Input: part model. Units: mm. Frame: model coordinates. Face numbers are marked on the shaded views. A direction names the side the tool comes from. Round coordinates to 2 decimals unless told otherwise and drop trailing zeros. Loops run counter-clockwise (first coordinate to the right, second up) from the corner with the lowest first, then second, coordinate; pieces in that order, holes last. Notation, with made-up numbers: M 84,46.25 L 98,46.25 A17 ccw 98,70.25 Z; hole C 35.5,47.5 d10. An arc over 180 degrees is marked long. Use one line per item in the form item = value. Start each with the question number.
Q1. Section query D-D, the plane y = 5.25. Output: boundary loops of the cut face in (x, z), and give its area (3 significant figures).
Q2. Mould query, pull axis Z, two halves, no side actions, for the marked faces 1, 2 and 3. Classes: pulls with the +Z half, pulls with the -Z half, needs draft (parallel to the pull), parting line crosses it, or undercut.
Q3. Section query A-A, the plane x = -13. Output: boundary loops of the cut face in (y, z), and give its area (3 significant figures).
Q4. Section query B-B, the plane z = 0. Output: boundary loops of the cut face in (x, y).
Q5. Access query for the marked faces 4, 5 and 6. Directions: +Z, -Z, +X, -X, +Y, -Y. A direction counts if a zero-diameter tool reaches every point of the face in a straight line with its end or side. Return the directions, or none.
Q6. Ray query, line 1 along Z through (x, y) = (-13.5, 1.25); line 2 along X through (y, z) = (-4.75, -0.75); line 3 along X through (y, z) = (-1.5, -1.25). Return the intervals inside material, ascending.
Q7. First-contact query: P1, Ø3, axis at x = -14, z = -0.5, coming from the -Y side; P2, Ø2, axis at y = 4.5, z = -4, coming from the +X side; P3, Ø1.5, axis at x = -4, y = 0.5, coming from the +Z side. Flat tips, straight axial feed; report the tip coordinate or a pass-through.
Q8. Section query C-C, the plane x = 8.5. Output: boundary loops of the cut face in (y, z), and give its area (3 significant figures).
Solid Edge part; units mm, degrees
sketch "Sketch1" plane through (10.8674, 0, 10.8674) normal (0, -1, 0) x (1, 0, 0)
  line L0 (-27.3674, -10.8674) -> (-27.3674, -4.3674)
  line L1 (-27.3674, -4.3674) -> (-19.3674, -4.3674)
  line L2 (-19.3674, -4.3674) -> (-19.3674, -6.4674)
  arc A0 (-19.3674, -6.4674) -> (-18.9674, -6.8674) centre (-18.9674, -6.4674) ccw
  line L3 (-18.9674, -6.8674) -> (5.6326, -6.8674)
  line L4 (5.6326, -6.8674) -> (5.6326, -10.8674)
revolve "RevolvedProtrusion1" add sketch "Sketch1" angle 360 about axis through (16.5, 0, 0) along (-1, 0, 0)
sketch "Sketch2" plane through (-16.5, 0, 0) normal (-1, 0, 0) x (0, 0, -1)
  line L0 (3.4641, 0) -> (1.7321, 3)
  line L1 (1.7321, 3) -> (-1.7321, 3)
  line L2 (-1.7321, 3) -> (-3.4641, 0)
  line L3 (-3.4641, 0) -> (-1.7321, -3)
  line L4 (-1.7321, -3) -> (1.7321, -3)
  line L5 (1.7321, -3) -> (3.4641, 0)
extrude "Cutout1" cut sketch "Sketch2" against normal blind 4
cosmetic_thread "Gänga" thread depth 20
properties material "Steel"
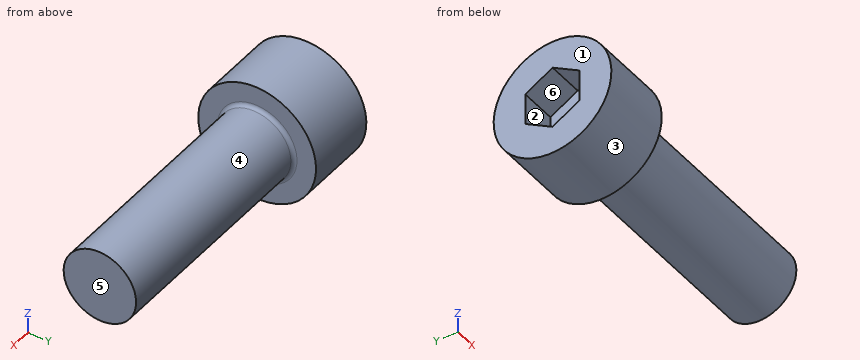
Results found:
q1.outline = M -16.5,-3.83 L -8.5,-3.83 L -8.5,3.83 L -16.5,3.83 Z
q1.area = 61.3 mm²
q2.face_1 = needs draft
q2.face_2 = undercut
q2.face_3 = parting line crosses it
q3.outline = C 0,0 d13; hole M -3,-1.73 L 0,-3.46 L 3,-1.73 L 3,1.73 L 0,3.46 L -3,1.73 Z
q3.area = 102 mm²
q4.outline = M -16.5,-6.5 L -8.5,-6.5 L -8.5,-4.4 A0.4 cw -8.1,-4 L 16.5,-4 L 16.5,4 L -8.1,4 A0.4 cw -8.5,4.4 L -8.5,6.5 L -16.5,6.5 L -16.5,3 L -12.5,3 L -12.5,-3 L -16.5,-3 Z
q5.face_4 = +X
q5.face_5 = +Z, -Z, +X, +Y, -Y
q5.face_6 = -X
q6.line_1 = -6.38 to -2.74, 2.74 to 6.38
q6.line_2 = -16.5 to -8.5
q6.line_3 = -12.5 to 16.5
q7.P1 = -6.5
q7.P2 = -8.5
q7.P3 = 4
q8.outline = C 0,0 d8
q8.area = 50.3 mm²
